```python
from build123d import *

# Parameters (mm, degrees)
F0_W     = 77.1000012755
F0_H     = 39.9000020698
F1_DEPTH = 30
F3_DEPTH = 30.001
F4_W     = 28.0499991495
F4_H     = 23.7000000197
F5_DEPTH = 10
F6_T     = -2.5
F7_DEPTH = 10


with BuildPart() as f1:
    # F0 (on Top) → F1 (new body)
    with BuildSketch(Plane.XY):
        with Locations((-9.7500011325, 9.3000004999)):
            Rectangle(F0_W, F0_H)
    extrude(amount=F1_DEPTH)

    # F2 (on face) → F3 (cut, through all)
    with BuildSketch(Plane.XY.offset(30)):
        Polygon((-48.3000017703, 29.2500015348), (-48.3000017703, -10.650000535), (-26.1000003666, 15.1500003412), (28.7999995053, 29.2500015348), align=None)
        Polygon((-21.0000015795, -2.250000136), (-48.3000017703, -10.650000535), (28.7999995053, -10.650000535), (28.7999995053, -2.250000136), align=None)
    extrude(amount=-F3_DEPTH, mode=Mode.SUBTRACT)

    # F4 (on face) → F5 (cut)
    with BuildSketch(Plane.YZ.offset(28.7999995053)):
        with Locations((11.7749994388, 15.000000014)):
            Rectangle(F4_W, F4_H)
    extrude(amount=-F5_DEPTH, mode=Mode.SUBTRACT)

    # F6 (hollow: no face is removed)
    offset(amount=F6_T, kind=Kind.INTERSECTION, mode=Mode.SUBTRACT)

    # F7 (cut): a face of the model
    f7_faces = [f1.faces().sort_by_distance(p)[0] for p in [
        (18.7999995053, 11.7749994388, 15.000000014),
    ]]
    extrude(f7_faces, amount=-F7_DEPTH, mode=Mode.SUBTRACT)


solid = f1.part
```
Input: part model. Units: mm. Frame: model coordinates. A direction names the side the tool comes from. Round coordinates to 2 decimals unless told otherwise and drop trailing zeros. Write each loop counter-clockwise with the first axis right and the second up, starting at its lowest first coordinate (ties: lowest second). Pieces come first, ordered by that corner, then holes. Notation, with made-up numbers: (15.25, -22) - (27.25, -22) arc R34 cw to (27.25, 16) - close; hole circle Ø3 at (-38.75, 53.25). An arc over 180 degrees is marked (long way). Write item = value, one per line.
(1) Access query for faces 4 (the flat face through (22, 25.8, 15)), 5 (the flat face through (21, 12, 3.15)), 6 (the flat face through (8.8, -1, 15)), 7 (the flat face through (-30.93, -2.69, 15.18)). Directions: +Z, -Z, +X, -X, +Y, -Y. A direction counts if a zero-diameter tool reaches every point of the face in a straight line with its end or side. Return the directions, or none.
Geometry check:
face_4 = +X, -X, -Y
face_5 = +X, -Y
face_6 = +X, +Y, -Y
face_7 = none
(2) Contact query for flat-ended pins moving along their axis: pin 1 Ø8 at (y, z) = (-0.5, 9.5) entering from -X; pin 2 Ø0.7 at (y, z) = (-1.5, 19.5) entering from +X; pin 3 Ø10.5 at (x, z) = (21.5, 9) entering from -Y. Output: stop coordinate, or through.
Geometry check:
pin_1 = -43.01
pin_2 = 8.8
pin_3 = 25.8
(3) Section query C-C on y = -1. Output: boundary loops of the cut face in (x, z), then the cut area to 3 significant figures.
Geometry check:
outline = (-40, 0) - (28.8, 0) - (28.8, 3.15) - (8.8, 3.15) - (8.8, 26.85) - (28.8, 26.85) - (28.8, 30) - (-40, 30) - close; hole (-36.7, 2.5) - (-25.44, 2.5) - (-25.44, 27.5) - (-36.7, 27.5) - close
area = 1,310 mm^2
(4) Material intervals for probe 1 along Z at (x, y) = (1.5, 2.5); probe 2 along Y at (x, z) = (-0.5, 4); probe 3 along Y at (x, z) = (3, 15), sorted ascending.
Geometry check:
probe_1 = 0 to 2.5, 27.5 to 30
probe_2 = -2.25 to 0.25, 19.14 to 21.72
probe_3 = -2.25 to 0.25, 20.04 to 22.62
(5) Section query A-A on z = 12.5. Output: boundary loops of the cut face in (x, y), then the cut area to 3 significant figures.
Geometry check:
outline = (-48.3, -10.65) - (-21, -2.25) - (8.8, -2.25) - (8.8, 0.25) - (-21.38, 0.25) - (-40.75, -5.71) - (-24.72, 12.92) - (8.8, 21.53) - (8.8, 24.11) - (-26.1, 15.15) - close; (15.37, 25.8) - (28.8, 25.8) - (28.8, 29.25) - close
area = 321 mm^2
(6) Section query D-D on x = 20.5. Output: boundary loops of the cut face in (y, z), then the cut area to 3 significant figures.
Geometry check:
outline = (-2.25, 0) - (27.12, 0) - (27.12, 30) - (-2.25, 30) - (-2.25, 26.85) - (25.8, 26.85) - (25.8, 3.15) - (-2.25, 3.15) - close
area = 216 mm^2
(7) Section query B-B on x = -5.5. Output: boundary loops of the cut face in (y, z).
Geometry check:
outline = (-2.25, 0) - (20.44, 0) - (20.44, 30) - (-2.25, 30) - close; hole (0.25, 2.5) - (17.86, 2.5) - (17.86, 27.5) - (0.25, 27.5) - close
(8) Pull-direction query (Y, two-part tool) for faces 1 (the flat face through (-9.053, 16.947, 15.175)), 2 (the flat face through (-2, 10, 0)), 3 (the flat face through (-1, -2.25, 15)); classes: +Y half, -Y half, draft (parallel to the pull), parting line (faces both ways), or undercut.
Geometry check:
face_1 = undercut
face_2 = draft
face_3 = -Y half
